Geometry check sheet. Reference: the model listing, model coordinates, mm. Round coordinates to 2 decimals unless told otherwise and drop trailing zeros. Order: outer loops, then holes, each group sorted by start corner. A loop starts at its lowest first (then second) coordinate and runs counter-clockwise, first axis right, second up.
(1) Sectioned sample at C-C (z = 2.45). Give the number of separate pieces and of enclosed holes in the cut face, plus the area to 3 significant figures.
(2) Sectioned sample at B-B (x = -5). Record the boundary of the cut face in (y, z).
(3) Sectioned sample at D-D (y = -19). Record the boundary of the cut face in (x, z).
(4) Go/stop test with flat-tipped pins: pin 1 (2.5 mm diameter, centred on x = 42, y = 0, fed in from -Z); pin 2 (2 mm diameter, centred on y = 42, z = 2.5, fed in from -X) (3 decimals); pin 3 (3 mm diameter, centred on x = 30.5, z = 2.5, fed in from -Y). Record where each tip stops, or that it passes through.
(5) Sectioned sample at A-A (y = 70). Record the boundary of the cut face in (x, z) (3 decimals).
(6) Material ranges on line 1 along Y through (x, z) = (0, 4.8); line 2 along X through (y, z) = (49.5, 3.15); line 3 along Y through (x, z) = (9, 2.6), recorded low to high.
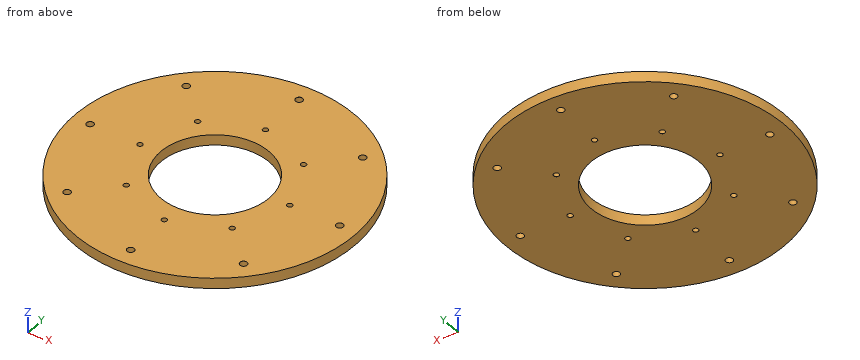
from build123d import *

# Parameters (mm, degrees)
SKETCH2_R                       = 80
SKETCH2_R_2                     = 31
BOSS_EXTRUDE1_DEPTH             = 6
F_4_0MM_DOWEL_HOLE1_D           = 4
F_4_0MM_DOWEL_HOLE1_CSINK_D     = 4.05
F_4_0MM_DOWEL_HOLE1_CSINK_ANGLE = 90
F_3_0MM_DOWEL_HOLE1_D           = 3
F_3_0MM_DOWEL_HOLE1_DEPTH       = 6
F_3_0MM_DOWEL_HOLE1_CSINK_D     = 3.05
F_3_0MM_DOWEL_HOLE1_CSINK_ANGLE = 90
F_3_0MM_DOWEL_HOLE1_TIP         = 0.901290929


with BuildPart() as part:
    # Sketch2 → Boss-Extrude1 (new body)
    with BuildSketch(Plane.XY):
        Circle(SKETCH2_R)
        Circle(SKETCH2_R_2, mode=Mode.SUBTRACT)
    extrude(amount=BOSS_EXTRUDE1_DEPTH)

    # Ø4.0mm Dowel Hole1 (through all)
    with Locations(Plane.XY.offset(6)):
        with Locations((0, 70), (-49.497474683, 49.497474683), (-70, 0), (-49.497474683, -49.497474683), (0, -70), (49.497474683, -49.497474683), (70, 0), (49.497474683, 49.497474683)):
            CounterSinkHole(F_4_0MM_DOWEL_HOLE1_D / 2, F_4_0MM_DOWEL_HOLE1_CSINK_D / 2, counter_sink_angle=F_4_0MM_DOWEL_HOLE1_CSINK_ANGLE)

    # Ø3.0mm Dowel Hole1
    with Locations(Plane(origin=(0, 0, 0), x_dir=(-1, 0, 0), z_dir=(0, 0, -1))):
        with Locations((-29.69848481, -29.69848481), (-42, 0), (-29.69848481, 29.69848481), (0, 42), (29.69848481, 29.69848481), (42, 0), (29.69848481, -29.69848481), (0, -42)):
            CounterSinkHole(F_3_0MM_DOWEL_HOLE1_D / 2, F_3_0MM_DOWEL_HOLE1_CSINK_D / 2, depth=F_3_0MM_DOWEL_HOLE1_DEPTH, counter_sink_angle=F_3_0MM_DOWEL_HOLE1_CSINK_ANGLE)
            with Locations((0, 0, -(F_3_0MM_DOWEL_HOLE1_DEPTH + F_3_0MM_DOWEL_HOLE1_TIP / 2))):  # 118° drill point
                Cone(0, F_3_0MM_DOWEL_HOLE1_D / 2, F_3_0MM_DOWEL_HOLE1_TIP, mode=Mode.SUBTRACT)


solid = part.part
Answer below:
1. separate pieces: 1
1. enclosed holes: 17
1. area: 16,900 mm2
2. outline: (-79.84, 0) - (-30.59, 0) - (-30.59, 6) - (-79.84, 6) - close; (30.59, 0) - (79.84, 0) - (79.84, 6) - (30.59, 6) - close
3. outline: (-77.71, 0) - (-24.49, 0) - (-24.49, 6) - (-77.71, 6) - close; (24.49, 0) - (77.71, 0) - (77.71, 6) - (24.49, 6) - close
4. pin 1: passes through
4. pin 2: stops at x = -68.695
4. pin 3: stops at y = -74.56
5. outline: (-38.73, 0) - (-2, 0) - (-2, 5.975) - (-2.025, 6) - (-38.73, 6) - close; (2, 0) - (38.73, 0) - (38.73, 6) - (2.025, 6) - (2, 5.975) - close
6. line 1: y = -80 to -72, -68 to -43.5, -40.5 to -31, 31 to 40.5, 43.5 to 68, 72 to 80
6. line 2: x = -62.85 to -51.5, -47.5 to 47.5, 51.5 to 62.85
6. line 3: y = -79.49 to -29.66, 29.66 to 79.49
